from build123d import *

# Parameters (mm, degrees)
SKETCH1_R           = 1.5
SKETCH1_R_2         = 1.75
SKETCH1_W           = 30
SKETCH1_H           = 5.5
BOSS_EXTRUDE1_DEPTH = 4
FILLET1_R           = 4
FILLET2_R           = 4
FILLET3_R           = 4
FILLET4_R           = 2.5


with BuildPart() as part:
    # Sketch1 → Boss-Extrude1 (new body)
    with BuildSketch(Plane(origin=(0, 0, 0), x_dir=(1, 0, 0), z_dir=(0, 1, 0))):
        Polygon((158.5, 0), (180, 0), (180, 10), (184, 10), (184, 0), (205, 0), (205, 112), (184, 112), (184, 102), (180, 102), (180, 112), (40, 112), (40, 102), (36, 102), (36, 112), (31, 112), (31, 116), (25, 116), (25, 112), (18.8632, 112), (0, 0), (36, 0), (36, 10), (40, 10), (40, 0), (95, 0), (95, 5.5), (108.5, 5.5), (108.5, 10), (107.3, 10), (107.3, 13), (108.5, 13), (108.5, 19.5), (111.5, 19.5), (111.5, 13), (112.7, 13), (112.7, 10), (111.5, 10), (111.5, 5.5), (125, 5.5), (125, 0), (155.5, 0), align=None)
        with Locations(Location((153.5, 89.25, 0), (0, 0, 270))):
            Circle(SKETCH1_R, mode=Mode.SUBTRACT)
        with Locations(Location((66.5, 89.25, 0), (0, 0, 270))):
            Circle(SKETCH1_R, mode=Mode.SUBTRACT)
        with Locations(Location((195, 104, 0), (0, 0, 270))):
            Circle(SKETCH1_R, mode=Mode.SUBTRACT)
        with Locations(Location((195, 84, 0), (0, 0, 270))):
            Circle(SKETCH1_R, mode=Mode.SUBTRACT)
        with Locations(Location((200, 94, 0), (0, 0, 270))):
            Circle(SKETCH1_R, mode=Mode.SUBTRACT)
        with Locations(Location((80, 15.5, 0), (0, 0, 270))):
            Circle(SKETCH1_R_2, mode=Mode.SUBTRACT)
        with Locations(Location((80, 25.5, 0), (0, 0, 270))):
            Circle(SKETCH1_R_2, mode=Mode.SUBTRACT)
        with Locations(Location((140, 15.5, 0), (0, 0, 270))):
            Circle(SKETCH1_R_2, mode=Mode.SUBTRACT)
        with Locations(Location((140, 25.5, 0), (0, 0, 270))):
            Circle(SKETCH1_R_2, mode=Mode.SUBTRACT)
        with Locations(Location((182, 26.5, 0), (0, 0, 270))):
            Circle(SKETCH1_R, mode=Mode.SUBTRACT)
        with Locations(Location((38, 16.5, 0), (0, 0, 270))):
            Circle(SKETCH1_R, mode=Mode.SUBTRACT)
        with Locations((110, 89.25)):
            Rectangle(SKETCH1_W, SKETCH1_H, mode=Mode.SUBTRACT)
    extrude(amount=BOSS_EXTRUDE1_DEPTH)

    # Fillet1
    fillet1_edges = [part.edges().sort_by_distance(p)[0] for p in [
        (0, 2, 0),
    ]]
    fillet(fillet1_edges, radius=FILLET1_R)

    # Fillet2
    fillet2_edges = [part.edges().sort_by_distance(p)[0] for p in [
        (205, 2, -112),
    ]]
    fillet(fillet2_edges, radius=FILLET2_R)

    # Fillet3
    fillet3_edges = [part.edges().sort_by_distance(p)[0] for p in [
        (205, 2, 0),
    ]]
    fillet(fillet3_edges, radius=FILLET3_R)

    # Fillet4
    fillet4_edges = [part.edges().sort_by_distance(p)[0] for p in [
        (25, 2, -116),
        (31, 2, -116),
    ]]
    fillet(fillet4_edges, radius=FILLET4_R)


solid = part.part
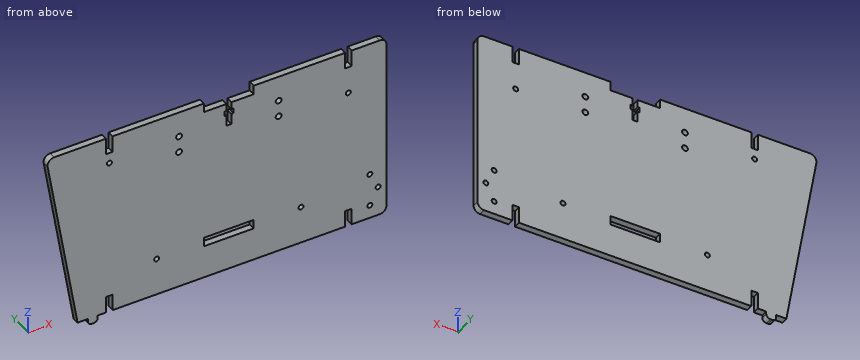
Source: CAD feature listing. Evaluate the final solid. Frame: model axes, mm. Give positions to 0.01 mm unless a question says otherwise; leave off trailing zeros. Write each loop counter-clockwise with the first axis right and the second up, starting at its lowest first coordinate (ties: lowest second). Pieces come first, ordered by that corner, then holes. Notation, with made-up numbers: M 9.25,-33.75 L 54.25,-33.75 A31 ccw 54.25,-0.75 Z; hole C 25,83 d9. An arc over 180 degrees is marked long. Answer as a JSON object with one key per item and string values.
Q1. Contact query for flat-ended pins moving along their axis: P1, Ø2.5, axis at x = 182, z = -26.5, coming from the -Y side; P2, Ø1.5, axis at x = 110.5, y = 2.5, coming from the +Z side; P3, Ø1.3, axis at x = 108, y = 1.5, coming from the -Z side; P4, Ø0.9, axis at y = 2, z = -12, coming from the -X side. Output: stop coordinate, or through.
Geometry check:
{"P1": "passes through", "P2": "stops at z = -19.5", "P3": "stops at z = -112", "P4": "stops at x = 1.95"}
Q2. Ray query, line 1 along Z through (x, y) = (80, 1.9); line 2 along Z through (x, y) = (66.5, 2.45); line 3 along X through (y, z) = (1.7, -26.5). Return the intervals inside material, ascending.
Geometry check:
{"line 1": "z = -112 to -27.25, -23.75 to -17.25, -13.75 to 0", "line 2": "z = -112 to -90.75, -87.75 to 0", "line 3": "x = 4.46 to 78.56, 81.44 to 138.56, 141.44 to 180.5, 183.5 to 205"}
Q3. Cut plane C-C, the plane z = -77. Return the cut outline in (x, y), then the cut area to 3 significant figures.
Geometry check:
{"outline": "M 12.97,0 L 205,0 L 205,4 L 12.97,4 Z", "area": "768 mm^2"}
Q4. Cut plane A-A, the plane x = 100. Return the cut outline in (y, z).
Geometry check:
{"outline": "M 0,-112 L 4,-112 L 4,-92 L 0,-92 Z; M 0,-86.5 L 4,-86.5 L 4,-5.5 L 0,-5.5 Z"}
Q5. Cut plane B-B, the plane x = 51.5. Return the cut outline in (y, z), then the cut area to 3 significant figures.
Geometry check:
{"outline": "M 0,-112 L 4,-112 L 4,0 L 0,0 Z", "area": "448 mm^2"}
